Read the model definition and answer for the solid it produces. Units are mm, in the model's axes. Round coordinates to 2 decimals unless told otherwise and drop trailing zeros. Write each loop counter-clockwise with the first axis right and the second up, starting at its lowest first coordinate (ties: lowest second). Pieces come first, ordered by that corner, then holes. Notation, with made-up numbers: (89.25, 10.5) -> (127.25, 10.5) arc R27 cw to (127.25, 45.5) -> close; hole circle Ø7 at (45.25, 14.5). An arc over 180 degrees is marked (long way). Return JSON: item names as keys, results as strings. Group by question number.
(1) Given pin 1 (2 mm diameter, centred on x = 31, y = 1.5, fed in from -Z); pin 2 (6 mm diameter, centred on x = -75, z = -5.5, fed in from -Y); pin 3 (5.5 mm diameter, centred on x = -170.18, z = 0, fed in from -Y), each flat-ended and moving along its own axis, determine where each tip first touches the part or whether it passes through.
(2) A cutting plane is placed at C-C on x = 135. Give the vertices of the cut face in (y, z), then the cut area to 3 significant figures.
(3) The mould has two halves that part along Z. Classify faces 1 (the flat face through (2.489, 0.928, -28.428)), 2 (the flat face through (2, 3.048, 0)), 3 (the flat face through (2.489, 0.928, 28.428)): released by +Z, released by -Z, zero draft, split by the parting line, or undercut.
(4) A cutting plane is placed at A-A on x = -102.5. Give the vertices of the cut face in (y, z), then the cut area to 3 significant figures.
(5) Straight lines are drawn through the part: line 1 (X direction, y = 2.3, z = 0); line 2 (Z direction, x = -170.18, y = 1.15); line 3 (Z direction, x = -31, y = 0.25). For each, find the intervals that lie inside material, in ascending order.
```python
from build123d import *

# Parameters (mm, degrees)
BOSS_EXTRUDE1_DEPTH = 177.8
CUT_EXTRUDE2_REACH  = 182.717
CUT_LOFT2_DEPTH     = 6.207121586
CUT_LOFT2_DRAFT     = -55.0003318
CUT_EXTRUDE4_REACH  = 182.717
CUT_LOFT3_START     = -177.779804528
CUT_LOFT3_DEPTH     = 355.618213607
FILLET7_R           = 2.54
FILLET8_R           = 2.54
CUT_EXTRUDE5_REACH  = 183.056
SKETCH19_R          = 2.4765


# Read off the part's stored shape, not the designer's step: Cut-Loft2, Cut-Loft3
with BuildPart() as part:
    # Sketch1 → Boss-Extrude1 (new, symmetric)
    with BuildSketch(Plane(origin=(0, 0, 0), x_dir=(0, 0, -1), z_dir=(1, 0, 0))):
        Polygon((0, 3.048), (25.4, 3.048), (35.052, -3.710403159), (33.303739022, -6.20717859), (24.438969291, 0), (0, 0), align=None)
    boss_extrude1 = extrude(amount=BOSS_EXTRUDE1_DEPTH, both=True)

    # Sketch4 → Cut-Extrude2 (cut, up to next)
    with BuildSketch(Plane(origin=(0, 13.979334982, -9.788435734), x_dir=(1, 0, 0), z_dir=(0, 0.8191520442889915, -0.5735764363510467)), mode=Mode.PRIVATE) as cut_extrude2_sk1:
        Polygon((-177.8, 30.841117278), (177.8, 24.949659112), (177.8, 30.841117278), align=None)
    cut_extrude2_tool1 = extrude(cut_extrude2_sk1.sketch, amount=-CUT_EXTRUDE2_REACH, mode=Mode.PRIVATE) & part.part
    cut_extrude2 = cut_extrude2_tool1.solids().sort_by_distance((59.266667, -2.584003, -33.443333))[0]
    add(cut_extrude2, mode=Mode.SUBTRACT)


with BuildPart() as cut_loft2_tool:
    # Cut-Loft2 outline → Cut-Loft2 (with draft: the straight prism first)
    with BuildSketch(Plane(origin=(-0.003265654, 0.761986004, 0), x_dir=(0.9999908164530384, 0.0042856749276558815, 0), z_dir=(0.0042856749276558815, -0.9999908164530384, 0))):
        Polygon((177.804898534, -24.919484646), (177.804898534, 0), (-177.798367166, 0), (-177.798367166, -24.438969291), align=None)
    extrude(amount=CUT_LOFT2_DEPTH)
    # Cut-Loft2: the draft: its side faces are tilted about the plane it starts from
    cut_loft2_sides = [cut_loft2_tool.faces().sort_by_distance(p)[0] for p in [
        (177.813300853, -1.579532292, -12.459742323),
        (0.013300853, -2.341532292, 0),
        (-177.786699148, -3.103532292, -12.219484645),
        (0.013300853, -2.341532292, -24.679226969),
    ]]
    draft(cut_loft2_sides, Plane(origin=(-0.003265654, 0.761986004, 0), x_dir=(0.9999908164530384, 0.0042856749276558815, 0), z_dir=(0.0042856749276558815, -0.9999908164530384, 0)), CUT_LOFT2_DRAFT)


with BuildPart() as part_1:
    add(part.part)

    # Cut-Loft2: cut by cut_loft2_tool
    add(cut_loft2_tool.part, mode=Mode.SUBTRACT)

    # Cut-Extrude4: up to this plane
    cut_extrude4_end = Plane(origin=(177.8, -1.579589295, -29.351869511), z_dir=(0.00428567492765589, -0.819144521567724, 0.5735711688849072))
    # Sketch12 → Cut-Extrude4 (cut, up to the surface)
    with BuildSketch(Plane(origin=(0, 13.979334982, -9.788435734), x_dir=(1, 0, 0), z_dir=(0, 0.8191520442889914, -0.5735764363510467)), mode=Mode.PRIVATE) as cut_extrude4_sk1:
        Polygon((-177.8, 30.841117278), (-50.8, 28.737025076), (-177.8, 24.949659112), align=None)
    cut_extrude4_tool1 = split(extrude(cut_extrude4_sk1.sketch, amount=-CUT_EXTRUDE4_REACH, mode=Mode.PRIVATE), bisect_by=cut_extrude4_end, keep=Keep.BOTH, mode=Mode.PRIVATE)
    cut_extrude4 = cut_extrude4_tool1.solids().sort_by_distance((-135.466667, -2.181717, -32.86881))[0]
    add(cut_extrude4, mode=Mode.SUBTRACT)

    # Mirror20: Boss-Extrude1 across plane
    add(boss_extrude1.mirror(Plane.XY))

    # Cut-Loft3 outline → Cut-Loft3 (cut)
    with BuildSketch(Plane(origin=(0, 0, 0), x_dir=(-0.004285667102275099, 0.999990816469807, -5.791138486653598e-06), z_dir=(0.9999899034999146, 0.0042856710149996365, 0.0013512668805631468)).offset(CUT_LOFT3_START)):
        Polygon((0.762004584, -2), (0.761850081, 24.679204437), (-5.720934875, 33.93758085), (-6.464848773, 35), (-8, 35), (-8, -2), align=None)
    extrude(amount=CUT_LOFT3_DEPTH, mode=Mode.SUBTRACT)

    # Mirror21: Cut-Extrude4 across plane
    add(cut_extrude4.mirror(Plane.XY), mode=Mode.SUBTRACT)

    # Mirror22: Cut-Extrude2 across plane
    add(cut_extrude2.mirror(Plane.XY), mode=Mode.SUBTRACT)

    # Fillet7
    fillet7_edges = [part_1.edges().sort_by_distance(p)[0] for p in [
        (-177.8, -1.579589295, -29.351869511),
        (-177.8, -1.579589295, 29.351869511),
    ]]
    fillet(fillet7_edges, radius=FILLET7_R)

    # Fillet8
    fillet8_edges = [part_1.edges().sort_by_distance(p)[0] for p in [
        (177.8, -0.955395437, -29.788934755),
        (177.8, -0.955395437, 29.788934755),
    ]]
    fillet(fillet8_edges, radius=FILLET8_R)

    # Cut-Extrude5: up to this plane
    cut_extrude5_end = Plane(origin=(177.8, 1.524, -24.919484646), z_dir=(0.004285674927655877, -0.9999908164530384, 0))
    # Sketch19 → Cut-Extrude5 (cut, up to the surface)
    with BuildSketch(Plane(origin=(0, 3.048, 0), x_dir=(1, 0, 0), z_dir=(0, 1, 0)), mode=Mode.PRIVATE) as cut_extrude5_sk1:
        with Locations(Location((-170.18, 0, 0), (0, 0, 270))):
            Circle(SKETCH19_R)
    cut_extrude5_tool1 = split(extrude(cut_extrude5_sk1.sketch, amount=-CUT_EXTRUDE5_REACH, mode=Mode.PRIVATE), bisect_by=cut_extrude5_end, keep=Keep.BOTH, mode=Mode.PRIVATE)
    add(cut_extrude5_tool1.solids().sort_by_distance((-170.18, 3.048, 0))[0], mode=Mode.SUBTRACT)


solid = part_1.part
```
Checks:
{
 "1": {"pin 1": "stops at z = -29.04", "pin 2": "stops at y = 0.43", "pin 3": "stops at y = 0.02"},
 "2": {"outline": "(-2.14, -29.83) -> (-0.74, -30.81) -> (3.05, -25.4) -> (3.05, 25.4) -> (-0.74, 30.81) -> (-2.14, 29.83) -> (1.34, 24.86) -> (1.34, -24.86) -> close", "area": "107 mm^2"},
 "3": {"face 1": "released by -Z", "face 2": "zero draft", "face 3": "released by +Z"},
 "4": {"outline": "(-3.85, -30.5) -> (-1.62, -32.07) -> (3.05, -25.4) -> (3.05, 25.4) -> (-1.62, 32.07) -> (-3.85, 30.5) -> (0.32, 24.54) -> (0.32, -24.54) -> close", "area": "178 mm^2"},
 "5": {"line 1": "x = -177.8 to -172.66, -167.7 to 177.8", "line 2": "z = -28.11 to -2.48, 2.48 to 28.11", "line 3": "z = -29.4 to -25.18, 25.18 to 29.4"}
}
